from build123d import *

# Parameters (mm, degrees)
BASE_FLANGE1_DEPTH      = 11
SKETCH5_R               = 4
SKETCH5_R_2             = 1.3
SKETCH5_R_3             = 1.05
CUT_EXTRUDE1_DEPTH      = 10
CUT_EXTRUDE2_DEPTH      = 45.273044847
CUT_EXTRUDE2_DEPTH_BACK = 45.273044847
SKETCH6_R               = 1.05
CUT_EXTRUDE3_DEPTH      = 10
FILLET1_R               = 2
EDGE_FLANGE1_DEPTH      = 44.34
FILLET2_R               = 2
FILLET2_OF_MIRROR1_R    = 2
BOSS_EXTRUDE2_DEPTH     = 2
FILLET4_R               = 2
SKETCH15_R              = 1.3
CUT_EXTRUDE5_DEPTH      = 2
CUT_EXTRUDE6_DEPTH      = 10
FILLET5_R               = 2


# Sheet-metal steps are written as plain solids
with BuildPart() as part:
    # Sketch1 → Base-Flange1 (new, symmetric)
    with BuildSketch(Plane.XY):
        with BuildLine():
            Line((-26.55, 32), (-26.55, 3.33))
            ThreePointArc((-26.55, 3.33), (-25.574665581, 0.975334419), (-23.22, 0))
            Line((-23.22, 0), (21.12, 0))
            ThreePointArc((21.12, 0), (23.474665581, 0.975334419), (24.45, 3.33))
            Line((24.45, 3.33), (24.45, 32))
            Line((24.45, 32), (26.45, 32))
            Line((26.45, 32), (26.45, 3.33))
            ThreePointArc((26.45, 3.33), (24.888879144, -0.438879144), (21.12, -2))
            Line((21.12, -2), (-23.22, -2))
            ThreePointArc((-23.22, -2), (-26.988879144, -0.438879144), (-28.55, 3.33))
            Line((-28.55, 3.33), (-28.55, 32))
            Line((-28.55, 32), (-26.55, 32))
        make_face()
    extrude(amount=BASE_FLANGE1_DEPTH, both=True)

    # Sketch5 → Cut-Extrude1 (cut)
    with BuildSketch(Plane(origin=(0, 0, 0), x_dir=(1, 0, 0), z_dir=(0, 1, 0))):
        with Locations(Location((3.95, 0, 0), (0, 0, 180))):
            Circle(SKETCH5_R)
        with Locations(Location((18.95, 8, 0), (0, 0, 180))):
            Circle(SKETCH5_R_2)
        with Locations(Location((18.95, -8, 0), (0, 0, 180))):
            Circle(SKETCH5_R_2)
        with Locations(Location((-16.05, -8, 0), (0, 0, 180))):
            Circle(SKETCH5_R_2)
        with Locations(Location((-16.05, 8, 0), (0, 0, 180))):
            Circle(SKETCH5_R_2)
        with Locations(Location((-4.05, 0, 0), (0, 0, 180))):
            Circle(SKETCH5_R_3)
        with Locations(Location((-1.706854249, 5.656854249, 0), (0, 0, 180))):
            Circle(SKETCH5_R_3)
        with Locations(Location((3.95, 8, 0), (0, 0, 180))):
            Circle(SKETCH5_R_3)
        with Locations(Location((9.606854249, 5.656854249, 0), (0, 0, 180))):
            Circle(SKETCH5_R_3)
        with Locations(Location((11.95, 0, 0), (0, 0, 180))):
            Circle(SKETCH5_R_3)
        with Locations(Location((9.606854249, -5.656854249, 0), (0, 0, 180))):
            Circle(SKETCH5_R_3)
        with Locations(Location((3.95, -8, 0), (0, 0, 180))):
            Circle(SKETCH5_R_3)
        with Locations(Location((-1.706854249, -5.656854249, 0), (0, 0, 180))):
            Circle(SKETCH5_R_3)
    extrude(amount=-CUT_EXTRUDE1_DEPTH, mode=Mode.SUBTRACT)

    # Sketch6 → Cut-Extrude2 (cut, two sides: drawn at the far end of the back side and taken through both)
    with BuildSketch(Plane(origin=(0, 0, 0), x_dir=(0, 0, -1), z_dir=(1, 0, 0)).offset(-CUT_EXTRUDE2_DEPTH_BACK)):
        with Locations((0, 21.5)):
            Circle(SKETCH6_R)
        with Locations((-5.656854249, 23.843145751)):
            Circle(SKETCH6_R)
        with Locations((-8, 29.5)):
            Circle(SKETCH6_R)
        with Locations((-5.656854249, 35.156854249)):
            Circle(SKETCH6_R)
        with Locations((0, 37.5)):
            Circle(SKETCH6_R)
        with Locations((5.656854249, 35.156854249)):
            Circle(SKETCH6_R)
        with Locations((8, 29.5)):
            Circle(SKETCH6_R)
        with Locations((5.656854249, 23.843145751)):
            Circle(SKETCH6_R)
        with BuildLine():
            Line((4.05, 32), (-4.05, 32))
            Line((-4.05, 32), (-4.05, 29.5))
            ThreePointArc((-4.05, 29.5), (0, 25.45), (4.05, 29.5))
            Line((4.05, 29.5), (4.05, 32))
        make_face()
    extrude(amount=CUT_EXTRUDE2_DEPTH + CUT_EXTRUDE2_DEPTH_BACK, mode=Mode.SUBTRACT)

    # Sketch7 → Cut-Extrude3 (cut)
    with BuildSketch(Plane.ZY.offset(28.55)):
        with BuildLine():
            Line((-5.5, 32), (5.5, 32))
            Line((5.5, 32), (5.5, 29.5))
            ThreePointArc((5.5, 29.5), (0, 24), (-5.5, 29.5))
            Line((-5.5, 29.5), (-5.5, 32))
        make_face()
    extrude(amount=-CUT_EXTRUDE3_DEPTH, mode=Mode.SUBTRACT)

    # Fillet1
    fillet1_edges = [part.edges().sort_by_distance(p)[0] for p in [
        (-27.55, 32, -11),
        (25.45, 32, -11),
        (-27.55, 32, -5.5),
        (-27.55, 32, 5.5),
        (-27.55, 32, 11),
        (25.45, 32, 11),
    ]]
    fillet(fillet1_edges, radius=FILLET1_R)

    # Edge-Flange1 section (across the edge) → Edge-Flange1 (add)
    with BuildSketch(Plane(origin=(-23.22, 0, 14.33), x_dir=(0, 0, -1), z_dir=(1, 0, 0))):
        with BuildLine():
            Line((-2, 3.33), (-2, 4.5))
            Line((-2, 4.5), (0, 4.5))
            Line((0, 4.5), (0, 3.33))
            ThreePointArc((0, 3.33), (0.975334419, 0.975334419), (3.33, 0))
            Line((3.33, 0), (3.33, -2))
            ThreePointArc((3.33, -2), (-0.438879144, -0.438879144), (-2, 3.33))
        make_face()
    edge_flange1 = extrude(amount=EDGE_FLANGE1_DEPTH)

    # Fillet2
    fillet2_edges = [part.edges().sort_by_distance(p)[0] for p in [
        (-23.22, 4.5, 15.33),
        (21.12, 4.5, 15.33),
    ]]
    fillet(fillet2_edges, radius=FILLET2_R)

    # Mirror1: Edge-Flange1 across plane
    add(edge_flange1.mirror(Plane.XY))

    # Fillet2 of Mirror1
    fillet2_of_mirror1_edges = [part.edges().sort_by_distance(p)[0] for p in [
        (-23.22, 4.5, -15.33),
        (21.12, 4.5, -15.33),
    ]]
    fillet(fillet2_of_mirror1_edges, radius=FILLET2_OF_MIRROR1_R)

    # Sketch14 → Boss-Extrude2 (add)
    with BuildSketch(Plane(origin=(26.45, 0, 0), x_dir=(0, 0, -1), z_dir=(1, 0, 0))):
        with BuildLine():
            Line((-11, 29.5), (-14, 29.5))
            ThreePointArc((-14, 29.5), (-13.228756555, 24.917424305), (-11, 20.839745962))
            Line((-11, 20.839745962), (-11, 29.5))
        make_face()
        with BuildLine():
            Line((-9.25, 29.5), (-11, 29.5))
            Line((-11, 29.5), (-11, 20.839745962))
            ThreePointArc((-11, 20.839745962), (0, 15.5), (11, 20.839745962))
            Line((11, 20.839745962), (11, 29.5))
            Line((11, 29.5), (9.25, 29.5))
            ThreePointArc((9.25, 29.5), (0, 20.25), (-9.25, 29.5))
        make_face()
        with BuildLine():
            Line((-14, 32), (-14, 29.5))
            Line((-14, 29.5), (-11, 29.5))
            Line((-11, 29.5), (-11, 30))
            ThreePointArc((-11, 30), (-10.414213562, 31.414213562), (-9, 32))
            Line((-9, 32), (-14, 32))
        make_face()
        with BuildLine():
            Line((-11, 30), (-11, 29.5))
            Line((-11, 29.5), (-9.25, 29.5))
            ThreePointArc((-9.25, 29.5), (-9.163535023, 30.761794708), (-8.905756565, 32))
            Line((-8.905756565, 32), (-9, 32))
            ThreePointArc((-9, 32), (-10.414213562, 31.414213562), (-11, 30))
        make_face()
        with BuildLine():
            Line((11, 29.5), (14, 29.5))
            Line((14, 29.5), (14, 32))
            Line((14, 32), (9, 32))
            ThreePointArc((9, 32), (10.414213562, 31.414213562), (11, 30))
            Line((11, 30), (11, 29.5))
        make_face()
        with BuildLine():
            Line((11, 29.5), (11, 20.839745962))
            ThreePointArc((11, 20.839745962), (13.228756555, 24.917424305), (14, 29.5))
            Line((14, 29.5), (11, 29.5))
        make_face()
        with BuildLine():
            ThreePointArc((8.905756565, 32), (9.163535023, 30.761794708), (9.25, 29.5))
            Line((9.25, 29.5), (11, 29.5))
            Line((11, 29.5), (11, 30))
            ThreePointArc((11, 30), (10.414213562, 31.414213562), (9, 32))
            Line((9, 32), (8.905756565, 32))
        make_face()
    extrude(amount=-BOSS_EXTRUDE2_DEPTH)

    # Fillet4
    fillet4_edges = [part.edges().sort_by_distance(p)[0] for p in [
        (25.45, 32, 14),
        (25.45, 32, -14),
    ]]
    fillet(fillet4_edges, radius=FILLET4_R)

    # Sketch15 → Cut-Extrude5 (cut)
    with BuildSketch(Plane(origin=(26.45, 0, 0), x_dir=(0, 0, -1), z_dir=(1, 0, 0))):
        with Locations((0, 18.5)):
            Circle(SKETCH15_R)
        with Locations((-7.778174593, 21.721825407)):
            Circle(SKETCH15_R)
        with Locations((-11, 29.5)):
            Circle(SKETCH15_R)
        with Locations((-7.778174593, 37.278174593)):
            Circle(SKETCH15_R)
        with Locations((0, 40.5)):
            Circle(SKETCH15_R)
        with Locations((7.778174593, 37.278174593)):
            Circle(SKETCH15_R)
        with Locations((11, 29.5)):
            Circle(SKETCH15_R)
        with Locations((7.778174593, 21.721825407)):
            Circle(SKETCH15_R)
    extrude(amount=-CUT_EXTRUDE5_DEPTH, mode=Mode.SUBTRACT)

    # Sketch16 → Cut-Extrude6 (cut)
    with BuildSketch(Plane.ZY.offset(-24.45)):
        with BuildLine():
            Line((-4.05, 29.5), (-5.5, 29.5))
            ThreePointArc((-5.5, 29.5), (0, 24), (5.5, 29.5))
            Line((5.5, 29.5), (4.05, 29.5))
            ThreePointArc((4.05, 29.5), (0, 25.45), (-4.05, 29.5))
        make_face()
        with BuildLine():
            Line((-4.05, 32), (-4.05, 29.5))
            Line((-4.05, 29.5), (4.05, 29.5))
            Line((4.05, 29.5), (4.05, 32))
            Line((4.05, 32), (4.898979486, 32))
            ThreePointArc((4.898979486, 32), (0, 35), (-4.898979486, 32))
            Line((-4.898979486, 32), (-4.05, 32))
        make_face()
        with BuildLine():
            ThreePointArc((-4.898979486, 32), (-5.347634392, 30.785615189), (-5.5, 29.5))
            Line((-5.5, 29.5), (-4.05, 29.5))
            Line((-4.05, 29.5), (-4.05, 32))
            Line((-4.05, 32), (-4.898979486, 32))
        make_face()
        with BuildLine():
            Line((-5.5, 32), (-5.5, 29.5))
            ThreePointArc((-5.5, 29.5), (-5.347634392, 30.785615189), (-4.898979486, 32))
            Line((-4.898979486, 32), (-5.5, 32))
        make_face()
        with BuildLine():
            Line((-5.5, 36.162581974), (-5.5, 32))
            Line((-5.5, 32), (-4.898979486, 32))
            ThreePointArc((-4.898979486, 32), (0, 35), (4.898979486, 32))
            Line((4.898979486, 32), (5.5, 32))
            Line((5.5, 32), (5.5, 36.162581974))
            Line((5.5, 36.162581974), (-5.5, 36.162581974))
        make_face()
        with BuildLine():
            Line((4.05, 29.5), (5.5, 29.5))
            ThreePointArc((5.5, 29.5), (5.347634392, 30.785615189), (4.898979486, 32))
            Line((4.898979486, 32), (4.05, 32))
            Line((4.05, 32), (4.05, 29.5))
        make_face()
        with BuildLine():
            ThreePointArc((4.898979486, 32), (5.347634392, 30.785615189), (5.5, 29.5))
            Line((5.5, 29.5), (5.5, 32))
            Line((5.5, 32), (4.898979486, 32))
        make_face()
    extrude(amount=-CUT_EXTRUDE6_DEPTH, mode=Mode.SUBTRACT)

    # Fillet5
    fillet5_edges = [part.edges().sort_by_distance(p)[0] for p in [
        (25.45, 32, 5.5),
        (25.45, 32, -5.5),
    ]]
    fillet(fillet5_edges, radius=FILLET5_R)


solid = part.part
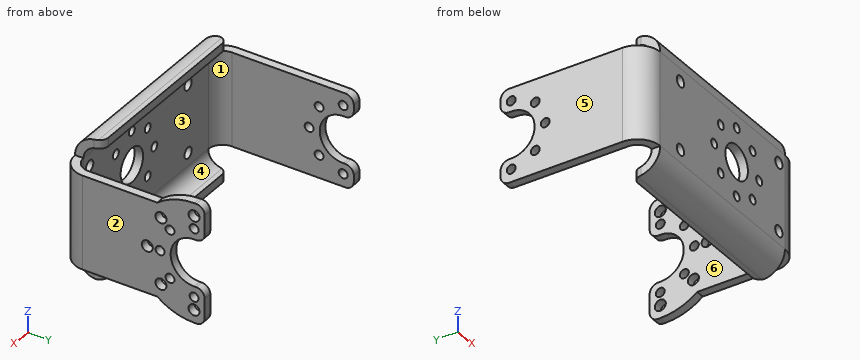
The model under review builds one solid part; all positions refer to its coordinate system, in mm. Face numbers are marked on the shaded views. A direction names the side the tool comes from. Round coordinates to 2 decimals unless told otherwise and drop trailing zeros. Loops run counter-clockwise (first coordinate to the right, second up) from the corner with the lowest first, then second, coordinate; pieces in that order, holes last. Notation, with made-up numbers: (67, 13) -> (120, 13) arc R23 ccw to (120, 47) -> close; hole circle Ø10 at (62.25, 43). An arc over 180 degrees is marked (long way). One line per question, with ' | ' between items. Start each with the question number.
Item 1: Add section B-B, the plane y = 12.5. Write out the cut boundary in (x, z), then the cut area to 3 significant figures.
Item 2: For pin 1 (10 mm diameter, centred on x = 1.5, z = -9.5, fed in from +Y); pin 2 (2.5 mm diameter, centred on y = 21.5, z = 0, fed in from +X); pin 3 (3.5 mm diameter, centred on y = 0.5, z = 15, fed in from -X); pin 4 (6 mm diameter, centred on x = -1.5, z = 4.5, fed in from +Y), all flat-tipped, find the tip position at first contact; note any pin that passes through.
Item 3: Wall thickness on line 1 along X through (y, z) = (7.5, -10); line 2 along Z through (x, y) = (3.95, -1.25); line 3 along Y through (x, z) = (-6, 3): over which ranges is each line inside the solid? List them lowest first. Write a range as [from, to].
Item 4: Add section C-C, the plane z = 2.5. Write out the cut boundary in (x, y).
Item 5: Draft analysis for pull direction X (two halves, no side actions). For the marked faces 3, 4, 5 and 6, state which applies: +X half, -X half, draft (parallel to the pull), parting line (faces both ways), or undercut.
Item 6: Machinability: for the marked faces 1 and 2, which of the approach directions +Z, -Z, +X, -X, +Y, -Y give a long, thin tool a straight path to every point of the face, cutting with its end or side? Answer none if there is none.
Item 7: Add section D-D, the plane x = 6. Write out the cut boundary in (y, z).
Item 8: Add section A-A, the plane x = -16.05. Write out the cut boundary in (y, z).
Return value:
1) outline: (-28.55, -11) -> (-26.55, -11) -> (-26.55, 11) -> (-28.55, 11) -> close; (24.45, -11) -> (26.45, -11) -> (26.45, 11) -> (24.45, 11) -> close | area: 88.0 mm2
2) pin 1: stops at y = 4.5 | pin 2: stops at x = 26.45 | pin 3: stops at x = -23.22 | pin 4: stops at y = 0
3) line 1: x = [-28.55, -26.55], [24.45, 26.45] | line 2: z = [-13.73, -9.05], [-6.95, -4], [4, 6.95], [9.05, 13.73] | line 3: y = [-2, 0]
4) outline: (-28.55, 3.33) arc R5.33 ccw to (-23.22, -2) -> (0.83, -2) -> (0.83, 0) -> (-23.22, 0) arc R3.33 cw to (-26.55, 3.33) -> (-26.55, 24.6) -> (-28.55, 24.6) -> close; (7.07, -2) -> (21.12, -2) arc R5.33 ccw to (26.45, 3.33) -> (26.45, 24.6) -> (24.45, 24.6) -> (24.45, 3.33) arc R3.33 cw to (21.12, 0) -> (7.07, 0) -> close
5) face 3: undercut | face 4: draft | face 5: -X half | face 6: undercut
6) face 1: +Z, -Z, +Y | face 2: +Z, -Z, +X, +Y, -Y
7) outline: (-2, -11) arc R5.33 ccw to (3.33, -16.33) -> (4.5, -16.33) -> (4.5, -14.33) -> (3.33, -14.33) arc R3.33 cw to (0, -11) -> (0, -3.43) -> (-2, -3.43) -> close; (-2, 3.43) -> (0, 3.43) -> (0, 11) arc R3.33 cw to (3.33, 14.33) -> (4.5, 14.33) -> (4.5, 16.33) -> (3.33, 16.33) arc R5.33 ccw to (-2, 11) -> close
8) outline: (-2, -11) arc R5.33 ccw to (3.33, -16.33) -> (4.5, -16.33) -> (4.5, -14.33) -> (3.33, -14.33) arc R3.33 cw to (0, -11) -> (0, -9.3) -> (-2, -9.3) -> close; (-2, -6.7) -> (0, -6.7) -> (0, 6.7) -> (-2, 6.7) -> close; (-2, 9.3) -> (0, 9.3) -> (0, 11) arc R3.33 cw to (3.33, 14.33) -> (4.5, 14.33) -> (4.5, 16.33) -> (3.33, 16.33) arc R5.33 ccw to (-2, 11) -> close
